Build history of the part. All positions in model axes, mm. A direction names the side the tool comes from. Give positions to 0.01 mm unless a question says otherwise; leave off trailing zeros. Order: outer loops, then holes, each group sorted by start corner. A loop starts at its lowest first (then second) coordinate and runs counter-clockwise, first axis right, second up. Notation, with made-up numbers: M -15,59 L 43,59 A23 cw 43,72 Z; hole C 5,30.5 d3. An arc over 180 degrees is marked long. One line per item, written item: value.
from build123d import *
from OCP.BRepFilletAPI import BRepFilletAPI_MakeChamfer

# Parameters (mm, degrees)
SKETCH1_W           = 40
SKETCH1_H           = 25
BOSS_EXTRUDE1_DEPTH = 30
SKETCH2_W           = 44
SKETCH2_H           = 29
BOSS_EXTRUDE2_DEPTH = 10
SKETCH3_W           = 40
SKETCH3_H           = 25
BOSS_EXTRUDE3_DEPTH = 14
SKETCH4_W           = 40
SKETCH4_H           = 25
CUT_EXTRUDE1_DEPTH  = 7
SKETCH5_R           = 4
SKETCH5_R_2         = 2.65
CUT_EXTRUDE2_DEPTH  = 3
SKETCH6_R           = 6
BOSS_EXTRUDE4_DEPTH = 10
CHAMFER1_SIZE       = 2
CHAMFER1_SIZE_2     = 6.974828888


with BuildPart() as part:
    # Sketch1 → Boss-Extrude1 (new body)
    with BuildSketch(Plane(origin=(0, 0, 0), x_dir=(1, 0, 0), z_dir=(0, 1, 0))):
        with Locations((20, 12.5)):
            Rectangle(SKETCH1_W, SKETCH1_H)
    extrude(amount=BOSS_EXTRUDE1_DEPTH)

    # Sketch2 → Boss-Extrude2 (add)
    with BuildSketch(Plane(origin=(0, 0, 0), x_dir=(1, 0, 0), z_dir=(0, 1, 0))):
        with Locations((20, 12.5)):
            Rectangle(SKETCH2_W, SKETCH2_H)
    extrude(amount=BOSS_EXTRUDE2_DEPTH)

    # Sketch3 → Boss-Extrude3 (add)
    with BuildSketch(Plane.XZ):
        with Locations((20, -12.5)):
            Rectangle(SKETCH3_W, SKETCH3_H)
    extrude(amount=BOSS_EXTRUDE3_DEPTH)

    # Sketch4 → Cut-Extrude1 (cut)
    with BuildSketch(Plane.XZ.offset(14)):
        with Locations((20, -12.5)):
            Rectangle(SKETCH4_W, SKETCH4_H)
    extrude(amount=-CUT_EXTRUDE1_DEPTH, mode=Mode.SUBTRACT)

    # Sketch5 → Cut-Extrude2 (cut)
    # profile 1 of 2: a face of its own
    with BuildSketch(Plane.XZ.offset(7)):
        with Locations(Location((6.5, -12.5, 0), (0, 0, 270))):
            Circle(SKETCH5_R)
        with Locations(Location((6.5, -12.5, 0), (0, 0, 270))):
            Circle(SKETCH5_R_2, mode=Mode.SUBTRACT)
    # profile 2 of 2: a face of its own
    with BuildSketch(Plane.XZ.offset(7)):
        with Locations(Location((33.5, -12.5, 0), (0, 0, 90))):
            Circle(SKETCH5_R)
        with Locations(Location((33.5, -12.5, 0), (0, 0, 90))):
            Circle(SKETCH5_R_2, mode=Mode.SUBTRACT)
    extrude(amount=-CUT_EXTRUDE2_DEPTH, mode=Mode.SUBTRACT)

    # Sketch6 → Boss-Extrude4 (add)
    with BuildSketch(Plane.XZ.offset(7)):
        with Locations(Location((20, -12.5, 0), (0, 0, 90))):
            Circle(SKETCH6_R)
    extrude(amount=BOSS_EXTRUDE4_DEPTH)

    # Chamfer1
    chamfer1_edges_1 = [part.edges().sort_by_distance(p)[0] for p in [
        (0, 0, -12.5),
    ]]
    chamfer1_side_1 = [part.faces().sort_by_distance(p)[0] for p in [
        (-0.04, 0, -12.5),
    ]]
    chamfer1_edges_2 = [part.edges().sort_by_distance(p)[0] for p in [
        (20, 0, -25),
    ]]
    chamfer1_side_2 = [part.faces().sort_by_distance(p)[0] for p in [
        (20, 0, -25.04),
    ]]
    chamfer1_edges_3 = [part.edges().sort_by_distance(p)[0] for p in [
        (40, 0, -12.5),
    ]]
    chamfer1_side_3 = [part.faces().sort_by_distance(p)[0] for p in [
        (40.04, 0, -12.5),
    ]]
    chamfer1_edges_4 = [part.edges().sort_by_distance(p)[0] for p in [
        (20, 0, 0),
    ]]
    chamfer1_side_4 = [part.faces().sort_by_distance(p)[0] for p in [
        (20, 0, 0.04),
    ]]
    chamfer1 = BRepFilletAPI_MakeChamfer(part.part.solid().wrapped)
    for e in chamfer1_edges_1:
        chamfer1.Add(CHAMFER1_SIZE - 0.0001, CHAMFER1_SIZE_2 - 0.0001, e.wrapped, chamfer1_side_1[0].wrapped)
    for e in chamfer1_edges_2:
        chamfer1.Add(CHAMFER1_SIZE - 0.0001, CHAMFER1_SIZE_2 - 0.0001, e.wrapped, chamfer1_side_2[0].wrapped)
    for e in chamfer1_edges_3:
        chamfer1.Add(CHAMFER1_SIZE - 0.0001, CHAMFER1_SIZE_2 - 0.0001, e.wrapped, chamfer1_side_3[0].wrapped)
    for e in chamfer1_edges_4:
        chamfer1.Add(CHAMFER1_SIZE - 0.0001, CHAMFER1_SIZE_2 - 0.0001, e.wrapped, chamfer1_side_4[0].wrapped)
    add(Compound.cast(chamfer1.Shape()), mode=Mode.REPLACE)  # a hair under: the kernel refuses the full size


solid = part.part
1) Drill centre lines: probe 1 along Z at (x, y) = (6, -5); probe 2 along X at (y, z) = (-5.3, -12.5); probe 3 along Y at (x, z) = (4.5, -15.5). Where is each one in solid material? Low to high. Write a range as from..to.
Check values:
probe 1: -25.57..-16.47, -15.1..-9.9, -8.53..0.57
probe 2: -0.48..2.5, 3.85..9.15, 10.5..29.5, 30.85..36.15, 37.5..40.48
probe 3: -4..30
2) Mould opens along Z. For faces 1 (the face through (30.87, -5.52, -12.84)), 2 (the face through (29.534, -5.521, -13.021)), 3 (the face through (20, 20, -25)), 4 (the face through (18.3, 10, 0.3)) say: released by +Z, released by -Z, zero draft, split by the parting line, or undercut.
Check values:
face 1: undercut
face 2: undercut
face 3: released by -Z
face 4: zero draft
3) Saw through at C-C, the plane y = 24.5. Write the cut outline in (x, z).
Check values:
outline: M 0,-25 L 40,-25 L 40,0 L 0,0 Z
4) Tool access for faces 5 (the face through (6, -7, -12)), 6 (the face through (24, -7, -18)), 7 (the face through (0, 20, -12)), 8 (the face through (20, 30, -13)): list every direction of +Z, -Z, +X, -X, +Y, -Y with a clear straight run to the whole face (end or side of a thin tool).
Check values:
face 5: +Z, -Z, -X, -Y
face 6: -Y
face 7: +Z, -Z, -X, +Y
face 8: +Z, -Z, +X, -X, +Y
5) Pin check, flat tips, straight feed: pin 1 (9 mm diameter, centred on x = 32.5, z = -10.5, fed in from -Y); pin 2 (10 mm diameter, centred on y = 19, z = -13, fed in from -X); pin 3 (1 mm diameter, centred on x = 22.5, y = 22.5, fed in from -Z); pin 4 (1.5 mm diameter, centred on y = -12, z = -4, fed in from +X). Stop position of each tip, or through.
Check values:
pin 1: y = -7
pin 2: x = 0
pin 3: z = -25
pin 4: through
